Read the model definition and answer for the solid it produces. Units are mm, in the model's axes. A direction names the side the tool comes from. Give positions to 0.01 mm unless a question says otherwise; leave off trailing zeros. Order: outer loops, then holes, each group sorted by start corner. A loop starts at its lowest first (then second) coordinate and runs counter-clockwise, first axis right, second up. Notation, with made-up numbers: (16, 12.5) - (38, 12.5) arc R21 cw to (38, 46.5) - close; hole circle Ø1 at (26, 75). An arc over 180 degrees is marked (long way). Use a Markdown table: item, result. Add a question column.
1. A cutting plane is placed at C-C on x = 59. Determine the outline of the cut face in (y, z) (1 decimal), and give its area (3 significant figures).
2. Which of the six approach directions +Z, -Z, +X, -X, +Y, -Y give full straight-line access (tool end or side, diameter ignored) to faces 4 (the flat face through (50, -5, 16.857)), 5 (the flat face through (61, -9.525, 30)), 6 (the flat face through (45, -5, 35.751))?
3. A cutting plane is placed at B-B on z = 37. Determine the outline of the cut face in (x, y) (3 decimals), and give its area (3 significant figures).
4. Consider L1, parallel to X at y = -0.25, z = 26; L2, parallel to Z at x = 44, y = -7.25; L3, parallel to Z at x = 48.5, y = -7.25. Determine where each line is inside the solid, lowest interval first.
5. A cutting plane is placed at A-A on x = 52. Determine the outline of the cut face in (y, z) (3 decimals).
6. For a pull along Z with two mould halves and no side action, classify faces 1 (the cylindrical face through (47.87, -4.7, 31.12)), 2 (the cylindrical face through (49.22, -4.83, 36.51)), 3 (the flat face through (63.267, -4.696, 12.779)) as released by +Z, released by -Z, zero draft, split by the parting line, or undercut.
7. Flat-ended cylindrical pins translate along their axes: P1, Ø2, axis at x = 56, y = -8, coming from the -Z side; P2, Ø1, axis at y = -7.5, z = 44, coming from the -X side; P3, Ø4, axis at x = 45, y = -4, coming from the +Z side. Find the tip coordinate at first contact, or state that the pin passes through.
```python
from build123d import *

# Parameters (mm, degrees)
SKETCH11_R     = 5.434276133
EXTRUDE5_DEPTH = 9.525
FILLET2_R      = 2.54
FILLET1_R      = 2.54
FILLET3_R      = 2.54


with BuildPart() as part:
    # Sketch11 → Extrude5 (new body)
    # profile 1 of 4: a face of its own
    with BuildSketch(Plane(origin=(0, 0, 0), x_dir=(1, 0, 0), z_dir=(0, 1, 0))):
        with BuildLine():
            Line((68.401879092, -7.643838899), (59.189110378, -16.856607613))
            Line((59.189110378, -16.856607613), (41.505666101, -16.856607613))
            ThreePointArc((41.505666101, -16.856607613), (41.271917597, -16.860911304), (41.038485938, -16.873816546))
            ThreePointArc((41.038485938, -16.873816546), (37.127788442, -26.414950032), (41.505666101, -35.750954012))
            Line((41.505666101, -35.750954012), (49.948049738, -35.750954012))
            Line((49.948049738, -35.750954012), (49.948049738, -52.195324003))
            ThreePointArc((49.948049738, -52.195324003), (68.401879092, -44.551497607), (76.045705488, -26.097668253))
            ThreePointArc((76.045705488, -26.097668253), (74.059139732, -16.110527774), (68.401879092, -7.643838899))
        make_face()
        with Locations(Location((49.948049738, -26.097668253, 0), (0, 0, 270))):
            Circle(SKETCH11_R, mode=Mode.SUBTRACT)
    # profile 2 of 4: a face of its own
    with BuildSketch(Plane(origin=(0, 0, 0), x_dir=(1, 0, 0), z_dir=(0, 1, 0))):
        with BuildLine():
            Line((68.401879092, -7.643838899), (59.189110378, -16.856607613))
            Line((59.189110378, -16.856607613), (41.505666101, -16.856607613))
            ThreePointArc((41.505666101, -16.856607613), (41.271917597, -16.860911304), (41.038485938, -16.873816546))
            ThreePointArc((41.038485938, -16.873816546), (37.127788442, -26.414950032), (41.505666101, -35.750954012))
            Line((41.505666101, -35.750954012), (49.948049738, -35.750954012))
            Line((49.948049738, -35.750954012), (49.948049738, -52.195324003))
            ThreePointArc((49.948049738, -52.195324003), (68.401879092, -44.551497607), (76.045705488, -26.097668253))
            ThreePointArc((76.045705488, -26.097668253), (74.059139732, -16.110527774), (68.401879092, -7.643838899))
        make_face()
        with Locations(Location((49.948049738, -26.097668253, 0), (0, 0, 270))):
            Circle(SKETCH11_R, mode=Mode.SUBTRACT)
    # profile 3 of 4: a face of its own
    with BuildSketch(Plane(origin=(0, 0, 0), x_dir=(1, 0, 0), z_dir=(0, 1, 0))):
        with BuildLine():
            Line((68.401879092, -7.643838899), (59.189110378, -16.856607613))
            Line((59.189110378, -16.856607613), (41.505666101, -16.856607613))
            ThreePointArc((41.505666101, -16.856607613), (41.271917597, -16.860911304), (41.038485938, -16.873816546))
            ThreePointArc((41.038485938, -16.873816546), (37.127788442, -26.414950032), (41.505666101, -35.750954012))
            Line((41.505666101, -35.750954012), (49.948049738, -35.750954012))
            Line((49.948049738, -35.750954012), (49.948049738, -52.195324003))
            ThreePointArc((49.948049738, -52.195324003), (68.401879092, -44.551497607), (76.045705488, -26.097668253))
            ThreePointArc((76.045705488, -26.097668253), (74.059139732, -16.110527774), (68.401879092, -7.643838899))
        make_face()
        with Locations(Location((49.948049738, -26.097668253, 0), (0, 0, 270))):
            Circle(SKETCH11_R, mode=Mode.SUBTRACT)
    # profile 4 of 4: a face of its own
    with BuildSketch(Plane(origin=(0, 0, 0), x_dir=(1, 0, 0), z_dir=(0, 1, 0))):
        with BuildLine():
            Line((68.401879092, -7.643838899), (59.189110378, -16.856607613))
            Line((59.189110378, -16.856607613), (41.505666101, -16.856607613))
            ThreePointArc((41.505666101, -16.856607613), (41.271917597, -16.860911304), (41.038485938, -16.873816546))
            ThreePointArc((41.038485938, -16.873816546), (37.127788442, -26.414950032), (41.505666101, -35.750954012))
            Line((41.505666101, -35.750954012), (49.948049738, -35.750954012))
            Line((49.948049738, -35.750954012), (49.948049738, -52.195324003))
            ThreePointArc((49.948049738, -52.195324003), (68.401879092, -44.551497607), (76.045705488, -26.097668253))
            ThreePointArc((76.045705488, -26.097668253), (74.059139732, -16.110527774), (68.401879092, -7.643838899))
        make_face()
        with Locations(Location((49.948049738, -26.097668253, 0), (0, 0, 270))):
            Circle(SKETCH11_R, mode=Mode.SUBTRACT)
    extrude(amount=-EXTRUDE5_DEPTH)

    # Fillet2
    fillet2_edges = [part.edges().sort_by_distance(p)[0] for p in [
        (59.189110378, -4.7625, 16.856607613),
        (49.948049738, -4.7625, 35.750954012),
    ]]
    fillet(fillet2_edges, radius=FILLET2_R)

    # Fillet1
    fillet1_edges = [part.edges().sort_by_distance(p)[0] for p in [
        (68.401879092, -4.7625, 7.643838899),
        (49.948049738, -4.7625, 52.195324003),
    ]]
    fillet(fillet1_edges, radius=FILLET1_R)

    # Fillet3
    fillet3_edges = [part.edges().sort_by_distance(p)[0] for p in [
        (41.038485938, -4.7625, 16.873816546),
        (41.505666101, -4.7625, 35.750954012),
    ]]
    fillet(fillet3_edges, radius=FILLET3_R)


solid = part.part
```
Output values:
| question | item | result |
|---|---|---|
| 1 | outline | (-9.5, 16.7) - (0, 16.7) - (0, 50.6) - (-9.5, 50.6) - close |
| 1 | area | 323 mm² |
| 2 | face 4 | -Z, -X, +Y, -Y |
| 2 | face 5 | +Z, -Z, +X, -X, -Y |
| 2 | face 6 | +Z, -X, +Y, -Y |
| 3 | outline | (49.596, -9.525) - (73.659, -9.525) - (73.659, 0) - (49.596, 0) - close |
| 3 | area | 229 mm² |
| 4 | L1 | 37.12 to 44.51, 55.38 to 76.05 |
| 4 | L2 | 16.86 to 35.75 |
| 4 | L3 | 16.86 to 20.86, 31.34 to 36 |
| 5 | outline | (-9.525, 16.857) - (0, 16.857) - (0, 21.066) - (-9.525, 21.066) - close; (-9.525, 31.13) - (0, 31.13) - (0, 52.011) - (-9.525, 52.011) - close |
| 6 | face 1 | undercut |
| 6 | face 2 | released by +Z |
| 6 | face 3 | released by -Z |
| 7 | P1 | z = 16.86 |
| 7 | P2 | x = 49.95 |
| 7 | P3 | z = 35.75 |
